Could you check a few things on this model? Use its own coordinates, in mm. Round coordinates to 2 decimals unless told otherwise and drop trailing zeros. Loops run counter-clockwise (first coordinate to the right, second up) from the corner with the lowest first, then second, coordinate; pieces in that order, holes last. Notation, with made-up numbers: M 4,-24 L 8,-24 A26 cw 8,5 Z; hole C 40.25,68.5 d7. An arc over 180 degrees is marked long. One line per item, written item: value. Start each with the question number.
Q1. I'm going to push flat-ended pins straight in: pin 1 Ø6 at (x, y) = (3.5, -19) entering from -Z; pin 2 Ø1 at (y, z) = (-16, -2) entering from +X; pin 3 Ø2 at (x, y) = (-16, -19.5) entering from -Z. Where does each tip first touch, or does it pass through?
Q2. Imagine slicing it at C-C (x = -16). Please give me the cut outline in (y, z), then the cut area to 3 significant figures.
Q3. Please list where these lines run through material, in increasing order: line 1 along Z through (x, y) = (-15, -15.5); line 2 along X through (y, z) = (-13.25, 26.5); line 3 along X through (y, z) = (-15.25, -3).
Q4. Imagine slicing it at A-A (y = -10.25). Please give me the cut outline in (x, z), then the cut area to 3 significant figures.
Q5. Imagine slicing it at B-B (z = 8). Please give me the cut outline in (x, y), then the cut area to 3 significant figures.
from build123d import *

# Parameters (mm, degrees)
F1_DEPTH = 25.4


with BuildPart() as f1:
    # F0 (on Front) → F1 (new body)
    with BuildSketch(Plane.XZ):
        with BuildLine():
            Line((-29.301182, 15.078336), (-8.798818, -20.4328))
            ThreePointArc((-8.798818, -20.4328), (0, -25.5128), (8.798818, -20.4328))
            Line((8.798818, -20.4328), (29.301182, 15.078336))
            ThreePointArc((29.301182, 15.078336), (29.301182, 25.238336), (20.502364, 30.318336))
            Line((20.502364, 30.318336), (-20.502364, 30.318336))
            ThreePointArc((-20.502364, 30.318336), (-29.301182, 25.238336), (-29.301182, 15.078336))
        make_face()
    extrude(amount=F1_DEPTH)


solid = f1.part
Report:
1. pin 1: stops at z = -25.5
1. pin 2: stops at x = 19.73
1. pin 3: stops at z = -9.69
2. outline: M -25.4,-7.96 L 0,-7.96 L 0,30.32 L -25.4,30.32 Z
2. area: 972 mm²
3. line 1: z = -9.69 to 30.32
3. line 2: x = -28.44 to 28.44
3. line 3: x = -18.86 to 18.86
4. outline: M -29.3,15.08 L -8.8,-20.43 A10.16 ccw 8.8,-20.43 L 29.3,15.08 A10.16 ccw 20.5,30.32 L -20.5,30.32 A10.16 ccw Z
4. area: 2,300 mm²
5. outline: M -25.21,-25.4 L 25.21,-25.4 L 25.21,0 L -25.21,0 Z
5. area: 1,280 mm²
